Here's how the part is built. I have some questions about the finished solid (model axes, mm). A direction names the side the tool comes from. Round coordinates to 2 decimals unless told otherwise and drop trailing zeros. Loops run counter-clockwise (first coordinate to the right, second up) from the corner with the lowest first, then second, coordinate; pieces in that order, holes last. Notation, with made-up numbers: M 9,-3 L 57,-3 A33 cw 57,26 Z; hole C 17,31 d5. An arc over 180 degrees is marked long. Use a Markdown table: item, result.
from build123d import *

# Parameters (mm, degrees)
BOSS_EXTRUDE2_DEPTH = 12
CUT_EXTRUDE1_DEPTH  = 8.5
SKETCH6_R           = 1.5
CUT_EXTRUDE2_DEPTH  = 8.5


with BuildPart() as part:
    # Sketch2 → Boss-Extrude2 (new body)
    with BuildSketch(Plane(origin=(0, 0, 0), x_dir=(0, 1, 0), z_dir=(0, 0, 1))):
        with BuildLine():
            Line((-36.78, -21.5), (36.78, -21.5))
            Line((36.78, -21.5), (36.78, 9.5))
            ThreePointArc((36.78, 9.5), (33.265281374, 17.985281374), (24.78, 21.5))
            Line((24.78, 21.5), (-24.78, 21.5))
            ThreePointArc((-24.78, 21.5), (-33.265281374, 17.985281374), (-36.78, 9.5))
            Line((-36.78, 9.5), (-36.78, -21.5))
        make_face()
    extrude(amount=BOSS_EXTRUDE2_DEPTH)

    # Sketch5 → Cut-Extrude1 (cut)
    with BuildSketch(Plane.XY.offset(12)):
        with BuildLine():
            Line((21.5, -35.78), (-8.5, -35.78))
            ThreePointArc((-8.5, -35.78), (-16.985281374, -32.265281374), (-20.5, -23.78))
            Line((-20.5, -23.78), (-20.5, 23.78))
            ThreePointArc((-20.5, 23.78), (-16.985281374, 32.265281374), (-8.5, 35.78))
            Line((-8.5, 35.78), (21.5, 35.78))
            Line((21.5, 35.78), (21.5, -35.78))
        make_face()
    extrude(amount=-CUT_EXTRUDE1_DEPTH, mode=Mode.SUBTRACT)

    # Sketch6 → Cut-Extrude2 (cut)
    with BuildSketch(Plane.XY.offset(3.5)):
        with Locations((1.5, -5.78)):
            Circle(SKETCH6_R)
        with BuildLine():
            Line((9.75, -33.78), (-6.75, -33.78))
            ThreePointArc((-6.75, -33.78), (-18, -22.53), (-6.75, -11.28))
            Line((-6.75, -11.28), (9.75, -11.28))
            ThreePointArc((9.75, -11.28), (21, -22.53), (9.75, -33.78))
        make_face()
    extrude(amount=-CUT_EXTRUDE2_DEPTH, mode=Mode.SUBTRACT)


solid = part.part
1. Imagine slicing it at A-A, the plane x = -1. Write out the boundary of the cut face in (y, z), then the cut area to 3 significant figures.
Answer sheet:
| item | result |
|---|---|
| outline | M -36.78,0 L -33.78,0 L -33.78,3.5 L -35.78,3.5 L -35.78,12 L -36.78,12 Z; M -11.28,0 L 36.78,0 L 36.78,12 L 35.78,12 L 35.78,3.5 L -11.28,3.5 Z |
| area | 196 mm2 |
2. Imagine slicing it at D-D, the plane z = 2. Write out the boundary of the cut face in (x, y), then the cut area to 3 significant figures.
Answer sheet:
| item | result |
|---|---|
| outline | M -21.5,-24.78 A12 ccw -9.5,-36.78 L 21.5,-36.78 L 21.5,36.78 L -9.5,36.78 A12 ccw -21.5,24.78 Z; hole M -6.75,-33.78 L 9.75,-33.78 A11.25 ccw 9.75,-11.28 L -6.75,-11.28 A11.25 ccw Z; hole C 1.5,-5.78 d3 |
| area | 2,330 mm2 |
3. Imagine slicing it at B-B, the plane y = -22.53. Write out the boundary of the cut face in (x, z).
Answer sheet:
| item | result |
|---|---|
| outline | M -21.5,0 L -18,0 L -18,3.5 L -20.5,3.5 L -20.5,12 L -21.5,12 Z; M 21,0 L 21.5,0 L 21.5,3.5 L 21,3.5 Z |
4. We'd pull the mould along X, two halves only. Please class faces 1 (the face through (1, 8, 3.5)), 2 (the face through (0.31, -6.69, 1.77)), 3 (the face through (-20.5, 0, 8)): +X half, -X half, draft (parallel to the pull), parting line (faces both ways), or undercut.
Answer sheet:
| item | result |
|---|---|
| face 1 | draft |
| face 2 | undercut |
| face 3 | +X half |
5. Imagine slicing it at C-C, the plane z = 7.25. Write out the boundary of the cut face in (x, y).
Answer sheet:
| item | result |
|---|---|
| outline | M -21.5,-24.78 A12 ccw -9.5,-36.78 L 21.5,-36.78 L 21.5,-35.78 L -8.5,-35.78 A12 cw -20.5,-23.78 L -20.5,23.78 A12 cw -8.5,35.78 L 21.5,35.78 L 21.5,36.78 L -9.5,36.78 A12 ccw -21.5,24.78 Z |
6. Which directions (+Z, -Z, +X, -X, +Y, -Y) give clear straight access to the entire face, cutting with the end or side of a thin tool? Please do faces 4 (the face through (2, -33.78, 2)), 5 (the face through (6, 35.78, 8)), 6 (the face through (21.5, 0, 2)).
Answer sheet:
| item | result |
|---|---|
| face 4 | +Z, -Z |
| face 5 | +Z, +X |
| face 6 | +Z, -Z, +X, +Y, -Y |
7. For pin 1 Ø12.5 at (x, y) = (10.5, -7.5) entering from +Z; pin 2 Ø5 at (y, z) = (0.5, 9) entering from +X, each with a flat end and sliding along its axis, tell me the tip position at first contact or that it passes through.
Answer sheet:
| item | result |
|---|---|
| pin 1 | z = 3.5 |
| pin 2 | x = -20.5 |
8. I need wall thicknesses on probe 1 along Y at (x, z) = (1.5, 2.55); probe 2 along Y at (x, z) = (8.5, 3); probe 3 along Y at (x, z) = (14, 5.75). Which ranges of each line are inside material? Lowest first, please. Write a range as from..to.
Answer sheet:
| item | result |
|---|---|
| probe 1 | -36.78..-33.78, -11.28..-7.28, -4.28..36.78 |
| probe 2 | -36.78..-33.78, -11.28..36.78 |
| probe 3 | -36.78..-35.78, 35.78..36.78 |
